Part model, mm, in its own coordinate system. Face numbers are marked on the shaded views. Round coordinates to 2 decimals unless told otherwise and drop trailing zeros. Write each loop counter-clockwise with the first axis right and the second up, starting at its lowest first coordinate (ties: lowest second). Pieces come first, ordered by that corner, then holes.
1) Saw through at A-A on x = 0. Write the cut outline in (y, z).
2) Saw through at D-D on y = -49.5. Write the cut outline in (x, z).
3) Saw through at C-C on z = 38.5. Write the cut outline in (x, y), and give its area (3 significant figures).
4) Flat gauge pins, fed straight in: pin 1 (0.5 mm diameter, centred on x = -110.5, z = 20, fed in from -Y); pin 2 (4 mm diameter, centred on x = 38, y = 43.5, fed in from +Z); pin 3 (2 mm diameter, centred on y = 35.5, z = 5.5, fed in from +X); pin 4 (12 mm diameter, centred on x = 118.5, z = 6.5, fed in from -Y). Where does each tip first touch, or does it go through?
5) Pull direction Y, two halves, no side cores. Call the marked faces 1 and 2: +Y half, -Y half, draft (parallel to the pull), parting line (faces both ways), or undercut.
6) Drill centre lines: L1, parallel to Y at x = 0, z = 4.4; L2, parallel to Z at x = -102, y = -107; L3, parallel to Y at x = -81.5, z = 20. Where is each one in solid material? Low to high.
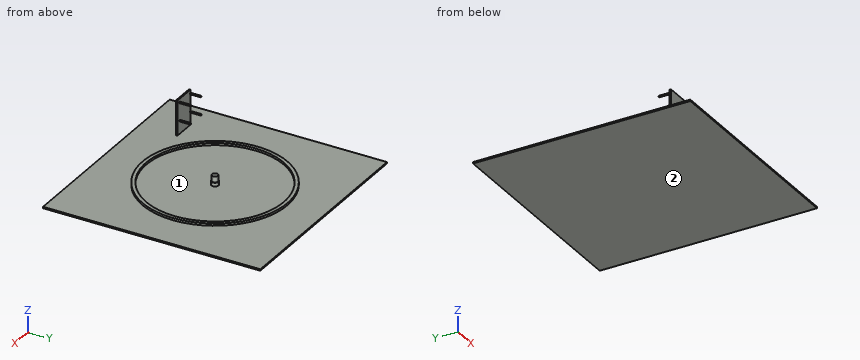
```python
from build123d import *

# Parameters (mm, degrees)
F0_W     = 300
F0_H     = 300
F0_W_2   = 30.8238497376
F0_H_2   = 2
F0_R     = 100
F0_R_2   = 94.9999988079
F0_R_3   = 5
F1_DEPTH = 2
F2_DEPTH = 15
F3_DEPTH = 5
F4_DEPTH = 50
F5_R     = 1
F6_DEPTH = 15
F7_R     = 5
F7_R_2   = 4
F8_DEPTH = 8


with BuildPart() as f1:
    # F0 (on Top) → F1 (new body)
    with BuildSketch(Plane.XY):
        Rectangle(F0_W, F0_H)
        with Locations((-94.5880751312, -99)):
            Rectangle(F0_W_2, F0_H_2, mode=Mode.SUBTRACT)
        Circle(F0_R, mode=Mode.SUBTRACT)
        Circle(F0_R)
        Circle(F0_R_2, mode=Mode.SUBTRACT)
        Circle(F0_R_2)
        Circle(F0_R_3, mode=Mode.SUBTRACT)
        with Locations((-94.5880751312, -99)):
            Rectangle(F0_W_2, F0_H_2)
    extrude(amount=F1_DEPTH)

    # F0 (on Top) → F2 (join)
    with BuildSketch(Plane.XY):
        Circle(F0_R_3)
    extrude(amount=F2_DEPTH)

    # F0 (on Top) → F3 (join)
    with BuildSketch(Plane.XY):
        Circle(F0_R)
        Circle(F0_R_2, mode=Mode.SUBTRACT)
    extrude(amount=F3_DEPTH)

    # F0 (on Top) → F4 (join)
    with BuildSketch(Plane.XY):
        with Locations((-94.5880751312, -99)):
            Rectangle(F0_W_2, F0_H_2)
    extrude(amount=F4_DEPTH)

    # F5 (on face) → F6 (join)
    with BuildSketch(Plane(origin=(0, -98, 0), x_dir=(-1, 0, 0), z_dir=(0, 1, 0))):
        with Locations((84.5761502624, 45)):
            Circle(F5_R)
        with BuildLine():
            Line((110, 44.0942674788), (110, 45.9057325212))
            ThreePointArc((110, 45.9057325212), (108.5761502624, 45), (110, 44.0942674788))
        make_face()
        with BuildLine():
            ThreePointArc((110, 44.0942674788), (110.4199066661, 44.4632736906), (110.5761502624, 45))
            ThreePointArc((110.5761502624, 45), (110.4199066661, 45.5367263094), (110, 45.9057325212))
            Line((110, 45.9057325212), (110, 44.0942674788))
        make_face()
        with BuildLine():
            Line((110, 19.0942674788), (110, 20.9057325212))
            ThreePointArc((110, 20.9057325212), (108.5761502624, 20), (110, 19.0942674788))
        make_face()
        with BuildLine():
            ThreePointArc((110.5761502624, 20), (110.4199066661, 20.5367263094), (110, 20.9057325212))
            Line((110, 20.9057325212), (110, 19.0942674788))
            ThreePointArc((110, 19.0942674788), (110.4199066661, 19.4632736906), (110.5761502624, 20))
        make_face()
        with Locations((84.5761502624, 20)):
            Circle(F5_R)
    extrude(amount=F6_DEPTH)

    # F7 (on face) → F8 (cut)
    with BuildSketch(Plane.XY.offset(15)):
        Circle(F7_R)
        Circle(F7_R_2, mode=Mode.SUBTRACT)
    extrude(amount=-F8_DEPTH, mode=Mode.SUBTRACT)


solid = f1.part
```
Completed:
1. outline: (-150, 0) - (150, 0) - (150, 2) - (100, 2) - (100, 5) - (95, 5) - (95, 2) - (5, 2) - (5, 7) - (4, 7) - (4, 15) - (-4, 15) - (-4, 7) - (-5, 7) - (-5, 2) - (-95, 2) - (-95, 5) - (-100, 5) - (-100, 2) - (-150, 2) - close
2. outline: (-150, 0) - (150, 0) - (150, 2) - (86.89, 2) - (86.89, 5) - (81.08, 5) - (81.08, 2) - (-81.08, 2) - (-81.08, 5) - (-86.89, 5) - (-86.89, 2) - (-150, 2) - close
3. outline: (-110, -100) - (-79.18, -100) - (-79.18, -98) - (-110, -98) - close
3. area: 61.6 mm2
4. pin 1: stops at y = -98
4. pin 2: stops at z = 2
4. pin 3: stops at x = 93.81
4. pin 4: stops at y = -150
5. face 1: undercut
5. face 2: draft
6. L1: y = -100 to -95, -5 to 5, 95 to 100
6. L2: z = 0 to 2
6. L3: y = -100 to -98
